For this review, take the finished solid that the model builds, in its own axes (mm). Round coordinates to 2 decimals unless told otherwise and drop trailing zeros. Write each loop counter-clockwise with the first axis right and the second up, starting at its lowest first coordinate (ties: lowest second). Pieces come first, ordered by that corner, then holes. Notation, with made-up numbers: (-9.5, -34.5) -> (32.5, -34.5) arc R20 cw to (32.5, -11.5) -> close; hole circle Ø9 at (23.25, 63). An arc over 180 degrees is marked (long way). Write item = value, one per line. Start each with the question number.
```python
from build123d import *

# Parameters (mm, degrees)
F0_W     = 5.08
F0_H     = 38.1
F1_DEPTH = 2.54
F2_SIZE2 = 4.905689
F2_SIZE  = 5.07999
F4_DEPTH = 25.4


# Not quite as in the source:
# - a fillet or chamfer is up to 0.001 mm smaller than in the source, because OpenCascade refuses the exact size


with BuildPart() as f1:
    # F0 (on Front) → F1 (new body)
    with BuildSketch(Plane.XZ):
        Rectangle(F0_W, F0_H)
    extrude(amount=F1_DEPTH)

    # F2 (size 5.08 and 4.905698976 in the source; OpenCascade refuses exactly that, so slightly less here)
    f2_edges = [f1.edges().sort_by_distance(p)[0] for p in [
        (2.54, -1.27, 19.05),
    ]]
    f2_side = f1.faces().sort_by_distance((0, -1.27, 19.05))[0]
    chamfer(f2_edges, length=F2_SIZE, length2=F2_SIZE2, reference=f2_side)

    # F3 (on face) → F4 (cut)
    with BuildSketch(Plane.XZ.offset(2.54)):
        with BuildLine():
            ThreePointArc((0, 4.318), (1.4368409794, 4.9131590206), (2.032, 6.35))
            ThreePointArc((2.032, 6.35), (-1.4368409794, 7.7868409794), (0, 4.318))
        make_face()
    extrude(amount=-F4_DEPTH, mode=Mode.SUBTRACT)


solid = f1.part
```
1. Wall thickness on L1, parallel to X at y = -0.55, z = 6.35; L2, parallel to Z at x = 1.35, y = -2.3; L3, parallel to Z at x = 0.5, y = -1.5: over which ranges is each line inside the solid? List them lowest first. Write a range as from..to.
2. Consider section A-A, the plane x = -0.8. Give the boundary of the cut face in (y, z), then the cut area to 3 significant figures.
3. Consider section B-B, the plane z = 5. Give the boundary of the cut face in (x, y).
Outcome:
q1.L1 = -2.54..-2.03, 2.03..2.54
q1.L2 = -19.05..4.83, 7.87..15.29
q1.L3 = -19.05..4.38, 8.32..16.11
q2.outline = (-2.54, -19.05) -> (0, -19.05) -> (0, 4.48) -> (-2.54, 4.48) -> close; (-2.54, 8.22) -> (0, 8.22) -> (0, 17.37) -> (-2.54, 17.37) -> close
q2.area = 83.0 mm2
q3.outline = (-2.54, -2.54) -> (-1.52, -2.54) -> (-1.52, 0) -> (-2.54, 0) -> close; (1.52, -2.54) -> (2.54, -2.54) -> (2.54, 0) -> (1.52, 0) -> close
